Design review of the part built by this model. Coordinates are the model's own, in mm. A direction names the side the tool comes from. Coordinates: 2 decimals unless noted, no trailing zeros. Loops run counter-clockwise (first coordinate to the right, second up) from the corner with the lowest first, then second, coordinate; pieces in that order, holes last. Notation, with made-up numbers: (75.5, 40) -> (113.5, 40) arc R37 cw to (113.5, 79) -> close; hole circle Ø2 at (86, 11). An arc over 180 degrees is marked (long way). One line per item, written item: value. Start each with the question number.
1. Draft analysis for pull direction X (two halves, no side actions). For faces 1 (the flat face through (-9.057, -13, 25)), 2 (the flat face through (-15.9, -9.7, 12.7)), 3 (the cylindrical face through (38.12, -21.58, 6.44)), 4 (the cylindrical face through (31.973, -18.334, 6.439)), state which applies: pulls with the +X half, pulls with the -X half, needs draft (parallel to the pull), parting line crosses it, or undercut.
2. Add section C-C on x = -26.5. Write out the cut boundary in (y, z).
3. Add section D-D on z = 15.5. Write out the cut boundary in (x, y), plus the area to 3 significant figures.
4. For probe 1 along X at (y, z) = (-17.25, 9); probe 2 along X at (y, z) = (-14, 6); probe 3 along X at (y, z) = (-19, 23), list the stretches that pass through material, from the lowest coordinate up.
5. Insertion check: pin 1 (3 mm diameter, centred on x = 8, z = 35, fed in from +Y); pin 2 (7.5 mm diameter, centred on x = 24.5, y = -10, fed in from +Z); pin 3 (12.5 mm diameter, centred on y = -15, z = 24, fed in from +X). Each pin has a flat end and moves straight along its axis. Give the tip position at first contact, or say it passes through.
6. Add section A-A on y = -16. Write out the cut boundary in (x, z).
7. Machinability: for faces 5 (the flat face through (16.343, -13, 25)), 6 (the cylindrical face through (-15.89, -15.13, 6.44)), which of the approach directions +Z, -Z, +X, -X, +Y, -Y give a long, thin tool a straight path to every point of the face, cutting with its end or side? Answer none if there is none.
```python
from build123d import *

# Parameters (mm, degrees)
F1_DEPTH  = 25.4
F2_R      = 12.7
F3_R      = 12.69999
F4_R      = 12.7
F5_R      = 12.69999
F6_R      = 12.7
F7_R      = 12.69999
F8_R      = 6.35
F9_DEPTH  = 25.4
F10_R     = 6.35
F11_DEPTH = 25.4
F12_R     = 6.35
F13_DEPTH = 25.4


# Not quite as in the source:
# - a fillet or chamfer is up to 0.001 mm smaller than in the source, because OpenCascade refuses the exact size


with BuildPart() as f1:
    # F0 (on Front) → F1 (new body)
    with BuildSketch(Plane.XZ):
        Polygon((-34.4568602741, 12.7), (-34.4568602741, 0), (41.7431397259, 0), (41.7431397259, 12.7), (16.3431397259, 12.7), (16.3431397259, 44.45), (-9.0568602741, 44.45), (-9.0568602741, 12.7), align=None)
    extrude(amount=F1_DEPTH)

    # F2
    f2_edges = [f1.edges().sort_by_distance(p)[0] for p in [
        (41.74314, -25.4, 6.35),
    ]]
    fillet(f2_edges, radius=F2_R)

    # F3 (radius 12.7 in the source; OpenCascade refuses exactly that, so slightly less here)
    f3_edges = [f1.edges().sort_by_distance(p)[0] for p in [
        (41.74314, 0, 6.35),
    ]]
    fillet(f3_edges, radius=F3_R)

    # F4
    f4_edges = [f1.edges().sort_by_distance(p)[0] for p in [
        (-34.45686, -25.4, 6.35),
    ]]
    fillet(f4_edges, radius=F4_R)

    # F5 (radius 12.7 in the source; OpenCascade refuses exactly that, so slightly less here)
    f5_edges = [f1.edges().sort_by_distance(p)[0] for p in [
        (-34.45686, 0, 6.35),
    ]]
    fillet(f5_edges, radius=F5_R)

    # F6
    f6_edges = [f1.edges().sort_by_distance(p)[0] for p in [
        (3.64314, -25.4, 44.45),
    ]]
    fillet(f6_edges, radius=F6_R)

    # F7 (radius 12.7 in the source; OpenCascade refuses exactly that, so slightly less here)
    f7_edges = [f1.edges().sort_by_distance(p)[0] for p in [
        (3.64314, 0, 44.45),
    ]]
    fillet(f7_edges, radius=F7_R)

    # F8 (on face) → F9 (cut)
    with BuildSketch(Plane.XY.offset(12.7)):
        with Locations((29.0431397259, -12.7)):
            Circle(F8_R)
    extrude(amount=-F9_DEPTH, mode=Mode.SUBTRACT)

    # F10 (on face) → F11 (cut)
    with BuildSketch(Plane.XY.offset(12.7)):
        with Locations((-21.7568602741, -12.7)):
            Circle(F10_R)
    extrude(amount=-F11_DEPTH, mode=Mode.SUBTRACT)

    # F12 (on face) → F13 (cut)
    with BuildSketch(Plane.YZ.offset(16.3431397259)):
        with Locations((-12.7, 31.75)):
            Circle(F12_R)
    extrude(amount=-F13_DEPTH, mode=Mode.SUBTRACT)


solid = f1.part
```
Worked answers:
1. face 1: pulls with the -X half
1. face 2: needs draft
1. face 3: pulls with the +X half
1. face 4: undercut
2. outline: (-24.48, 0) -> (-16.92, 0) -> (-16.92, 12.7) -> (-24.48, 12.7) -> close; (-8.48, 0) -> (-0.92, 0) -> (-0.92, 12.7) -> (-8.48, 12.7) -> close
3. outline: (-9.06, -25.4) -> (16.34, -25.4) -> (16.34, 0) -> (-9.06, 0) -> close
3. area: 645 mm²
4. probe 1: x = -33.61 to -26.19, -17.33 to 24.61, 33.47 to 40.9
4. probe 2: x = -34.39 to -27.97, -15.54 to 22.83, 35.26 to 41.68
4. probe 3: x = -9.06 to 16.34
5. pin 1: stops at y = -0.12
5. pin 2: stops at z = 12.7
5. pin 3: stops at x = 16.34
6. outline: (-34.02, 0) -> (-27.18, 0) -> (-27.18, 12.7) -> (-34.02, 12.7) -> close; (-16.33, 0) -> (23.62, 0) -> (23.62, 12.7) -> (16.34, 12.7) -> (16.34, 26.32) -> (-9.06, 26.32) -> (-9.06, 12.7) -> (-16.33, 12.7) -> close; (-9.06, 37.18) -> (16.34, 37.18) -> (16.34, 44.01) -> (-9.06, 44.01) -> close; (34.47, 0) -> (41.31, 0) -> (41.31, 12.7) -> (34.47, 12.7) -> close
7. face 5: +Z, +X, +Y, -Y
7. face 6: +Z, -Z
